```python
from build123d import *

# Parameters (mm, degrees)
F1_DEPTH = 152.4
F0_W     = 919.2846153846
F0_H     = 19.05
F2_DEPTH = 152.4
F3_DEPTH = 152.4


with BuildPart() as f1:
    # F0 (on Front) → F1 (new body)
    with BuildSketch(Plane.XZ):
        Polygon((938.3346153846, 19.05), (938.3346153846, 0), (957.3846153846, 0), (957.3846153846, 609.6), (938.3346153846, 609.6), align=None)
    extrude(amount=F1_DEPTH)

    # F0 (on Front) → F2 (join, through all)
    with BuildSketch(Plane.XZ):
        with Locations((478.6923076923, 9.525)):
            Rectangle(F0_W, F0_H)
    extrude(amount=F2_DEPTH)

    # F0 (on Front) → F3 (join, through all)
    with BuildSketch(Plane.XZ):
        Polygon((0, 609.6), (0, 0), (19.05, 0), (19.05, 19.05), (19.05, 609.6), align=None)
    extrude(amount=F3_DEPTH)


solid = f1.part
```
Source: CAD feature listing. Evaluate the final solid. Frame: model axes, mm. A direction names the side the tool comes from. Coordinates: 2 decimals unless noted, no trailing zeros. Write each loop counter-clockwise with the first axis right and the second up, starting at its lowest first coordinate (ties: lowest second). Pieces come first, ordered by that corner, then holes. Notation, with made-up numbers: M -13.75,29.25 L 40.25,29.25 A22 cw 40.25,57.25 Z; hole C 58.5,39.5 d8. An arc over 180 degrees is marked long. Answer as a JSON object with one key per item and string values.
1. Cut plane C-C on x = 371.5. Output: boundary loops of the cut face in (y, z), plus the area to 3 significant figures.
Evaluation:
{"outline": "M -152.4,0 L 0,0 L 0,19.05 L -152.4,19.05 Z", "area": "2,900 mm^2"}
2. Access query for faces 1 (the flat face through (0, -75, 309)), 2 (the flat face through (472, -75, 19.05)). Directions: +Z, -Z, +X, -X, +Y, -Y. A direction counts if a zero-diameter tool reaches every point of the face in a straight line with its end or side. Return the directions, or none.
Evaluation:
{"face 1": "+Z, -Z, -X, +Y, -Y", "face 2": "+Z, +Y, -Y"}
3. Cut plane A-A on z = 355. Output: boundary loops of the cut face in (x, y).
Evaluation:
{"outline": "M 0,-152.4 L 19.05,-152.4 L 19.05,0 L 0,0 Z; M 938.33,-152.4 L 957.38,-152.4 L 957.38,0 L 938.33,0 Z"}
4. Cut plane B-B on y = -68. Output: boundary loops of the cut face in (x, z).
Evaluation:
{"outline": "M 0,0 L 957.38,0 L 957.38,609.6 L 938.33,609.6 L 938.33,19.05 L 19.05,19.05 L 19.05,609.6 L 0,609.6 Z"}
5. Contact query for a flat-ended pin moving along its axis: P1, Ø3, axis at x = 847.5, y = -112, coming from the +Z side. Output: stop coordinate, or through.
Evaluation:
{"P1": "z = 19.05"}
6. Ray query, L1, parallel to X at y = -54.5, z = 85; L2, parallel to Z at x = 224.5, y = -82.5. Return the intervals inside material, ascending.
Evaluation:
{"L1": "0 to 19.05, 938.33 to 957.38", "L2": "0 to 19.05"}
7. Draft query along X for faces 3 (the flat face through (938.335, -75, 318)), 4 (the flat face through (957.385, -75, 301)), 5 (the flat face through (264, 0, 13)). Return one class per face: released by +X, released by -X, zero draft, split by the parting line, or undercut.
Evaluation:
{"face 3": "undercut", "face 4": "released by +X", "face 5": "zero draft"}
